Geometry check sheet. Reference: the model listing, model coordinates, mm. A direction names the side the tool comes from. Coordinates: 2 decimals unless noted, no trailing zeros. Loops run counter-clockwise (first coordinate to the right, second up) from the corner with the lowest first, then second, coordinate; pieces in that order, holes last. Notation, with made-up numbers: (53, 10.5) - (60, 10.5) arc R20 cw to (60, 33.5) - close; hole circle Ø1 at (88.5, -16). An arc over 180 degrees is marked (long way). Write each question's results on one line, items separated by ' | '. Start each with the question number.
(1) Sectioned sample at D-D (z = 6). Enter the section's corners in (x, y) (3 decimals), plus the area to 3 significant figures.
(2) Mould release check, pull along Z, two halves, no side actions. Record for faces 4 (the face through (10, 0, 40.195)), 5 (the face through (0, 30, 7)), 6 (the face through (3, 22, 26.524)): pulls with the +Z half, pulls with the -Z half, needs draft (parallel to the pull), parting line crosses it, or undercut.
(3) Go/stop test with flat-tipped pins: pin 1 Ø5.5 at (x, z) = (3.5, 8.5) entering from +Y; pin 2 Ø1 at (x, z) = (4, 0) entering from +Y; pin 3 Ø4.5 at (x, z) = (9.5, 25) entering from +Y (3 decimals); pin 4 Ø5 at (x, y) = (10, 30.5) entering from -Z. Record where each tip stops, or that it passes through.
(4) Access from +Z, -Z, +X, -X, +Y, -Y to the whole of each face (thin tool, end or side, straight path). Record for faces 1 (the face through (12.509, 0, 36)), 2 (the face through (7.66, 0, 36)), 3 (the face through (3, 4.108, 15)).
(5) Sectioned sample at C-C (y = 15.5). Enter the section's corners in (x, z).
(6) Material ranges on probe 1 along Y at (x, z) = (5, 21) (3 decimals); probe 2 along Z at (x, y) = (2.5, 11); probe 3 along Z at (x, y) = (2, 8.5), recorded low to high.
(7) Sectioned sample at A-A (z = 22.5). Enter the section's corners in (x, y) (3 decimals), plus the area to 3 significant figures.
(8) Sectioned sample at B-B (x = 10.75). Enter the section's corners in (y, z) (3 decimals).
from build123d import *

# Parameters (mm, degrees)
SKETCH2_R           = 2.54
BOSS_EXTRUDE1_DEPTH = 5.08
SKETCH2_3_W         = 43.072058764
SKETCH2_3_H         = 3.81
BOSS_EXTRUDE2_DEPTH = 14.224
SKETCH3_R           = 1.40634392
CUT_EXTRUDE1_DEPTH  = 60.360259481
SKETCH4_W           = 4.849530786
SKETCH4_H           = 3.81
BOSS_EXTRUDE3_DEPTH = 7.62
SKETCH5_R           = 1.38768984
CUT_EXTRUDE2_DEPTH  = 64.860340465


with BuildPart() as part:
    # Sketch2 → Boss-Extrude1 (new body)
    with BuildSketch(Plane(origin=(0, 0, 0), x_dir=(0, 0, -1), z_dir=(1, 0, 0))):
        Polygon((-32.574690201, 1.905), (-32.574690201, 49.446642672), (10.497368563, 35.924444265), (10.497368563, 1.905), align=None)
        with Locations((5.166357723, 10.6934)):
            Circle(SKETCH2_R, mode=Mode.SUBTRACT)
        with Locations((-28.852153042, 37.629948803)):
            Circle(SKETCH2_R, mode=Mode.SUBTRACT)
        Polygon((-1.581280818, 35.349430166), (-1.581280818, 4.108230491), (-28.317741421, 4.108230491), align=None, mode=Mode.SUBTRACT)
        Polygon((-26.524187902, 32.381969715), (-26.524187902, 10.6934), (-7.962941991, 32.381969715), align=None, mode=Mode.SUBTRACT)
    extrude(amount=BOSS_EXTRUDE1_DEPTH)

    # Sketch2_3 → Boss-Extrude2 (add)
    with BuildSketch(Plane(origin=(0, 0, 0), x_dir=(0, 0, -1), z_dir=(1, 0, 0))):
        with Locations((-11.038660819, 0)):
            Rectangle(SKETCH2_3_W, SKETCH2_3_H)
    extrude(amount=BOSS_EXTRUDE2_DEPTH)

    # Sketch3 → Cut-Extrude1 (cut, through all)
    with BuildSketch(Plane(origin=(0, 1.905, 0), x_dir=(1, 0, 0), z_dir=(0, 1, 0))):
        with Locations(Location((8.034839411, -3.04906194, 0), (0, 0, 270))):
            Circle(SKETCH3_R)
    extrude(amount=-CUT_EXTRUDE1_DEPTH, mode=Mode.SUBTRACT)

    # Sketch4 → Boss-Extrude3 (add)
    with BuildSketch(Plane.XY.offset(32.574690201)):
        with Locations((10.0846687, 0)):
            Rectangle(SKETCH4_W, SKETCH4_H)
    extrude(amount=BOSS_EXTRUDE3_DEPTH)

    # Sketch5 → Cut-Extrude2 (cut, through all)
    with BuildSketch(Plane(origin=(0, 1.905, 0), x_dir=(1, 0, 0), z_dir=(0, 1, 0))):
        with Locations(Location((10.158864626, -37.143001749, 0), (0, 0, 270))):
            Circle(SKETCH5_R)
    extrude(amount=-CUT_EXTRUDE2_DEPTH, mode=Mode.SUBTRACT)


solid = part.part
Outcome:
1) outline: (0, -1.905) - (14.224, -1.905) - (14.224, 1.905) - (5.08, 1.905) - (5.08, 4.108) - (0, 4.108) - close; (0, 30.186) - (5.08, 30.186) - (5.08, 41.104) - (0, 41.104) - close | area: 121 mm2
2) face 4: pulls with the +Z half | face 5: needs draft | face 6: undercut
3) pin 1: stops at y = 42.75 | pin 2: stops at y = 39.38 | pin 3: stops at y = 1.905 | pin 4: passes through
4) face 1: +Z, +X, +Y, -Y | face 2: +Z, -X, +Y, -Y | face 3: +X, -X
5) outline: (0, -10.5) - (5.08, -10.5) - (5.08, 1.58) - (0, 1.58) - close; (0, 18.57) - (5.08, 18.57) - (5.08, 22.41) - (0, 22.41) - close; (0, 26.52) - (5.08, 26.52) - (5.08, 32.57) - (0, 32.57) - close
6) probe 1: y = -1.905 to 4.108, 12.659 to 17.148, 32.382 to 45.813 | probe 2: z = -10.5 to -7.69, -2.64 to 1.58, 22.42 to 26.26, 26.52 to 32.57 | probe 3: z = -10.5 to -6.45, -3.89 to 1.58, 24.56 to 32.57
7) outline: (0, -1.905) - (14.224, -1.905) - (14.224, 1.905) - (5.08, 1.905) - (5.08, 4.108) - (0, 4.108) - close; (0, 10.906) - (5.08, 10.906) - (5.08, 15.396) - (0, 15.396) - close; (0, 32.382) - (5.08, 32.382) - (5.08, 46.284) - (0, 46.284) - close | area: 159 mm2
8) outline: (-1.905, -10.497) - (1.905, -10.497) - (1.905, 35.888) - (-1.905, 35.888) - close; (-1.905, 38.398) - (1.905, 38.398) - (1.905, 40.195) - (-1.905, 40.195) - close
